Design review of the part built by this model. Coordinates are the model's own, in mm. Coordinates: 2 decimals unless noted, no trailing zeros. Write each loop counter-clockwise with the first axis right and the second up, starting at its lowest first coordinate (ties: lowest second). Pieces come first, ordered by that corner, then holes.
Solid Edge part; units mm, degrees
sketch "Sketch1" plane through (0, 0, 0) normal (0, -1, 0) x (1, 0, 0)
  line L0 (-7.62, -8.0821) -> (-7.62, -17.3179)
  line L1 (-7.62, -17.3179) -> (-12.7, -17.3179)
  line L2 (-12.7, -17.3179) -> (-12.7, -25.4)
  line L3 (-12.7, -25.4) -> (-4.6179, -25.4)
  line L4 (-4.6179, -20.32) -> (-4.6179, -25.4)
  line L5 (4.6179, -20.32) -> (-4.6179, -20.32)
  line L6 (4.6179, -25.4) -> (4.6179, -20.32)
  line L7 (4.6179, -25.4) -> (12.7, -25.4)
  line L8 (12.7, -25.4) -> (12.7, -17.3179)
  line L9 (12.7, -17.3179) -> (7.62, -17.3179)
  line L10 (7.62, -17.3179) -> (7.62, -8.0821)
  line L11 (7.62, -8.0821) -> (12.7, -8.0821)
  line L12 (12.7, -8.0821) -> (12.7, 0)
  line L13 (12.7, 8.0821) -> (12.7, 0)
  line L14 (7.62, 8.0821) -> (12.7, 8.0821)
  line L15 (7.62, 17.3179) -> (7.62, 8.0821)
  line L16 (12.7, 17.3179) -> (7.62, 17.3179)
  line L17 (12.7, 25.4) -> (12.7, 17.3179)
  line L18 (4.6179, 25.4) -> (12.7, 25.4)
  line L19 (4.6179, 25.4) -> (4.6179, 20.32)
  line L20 (4.6179, 20.32) -> (-4.6179, 20.32)
  line L21 (-4.6179, 20.32) -> (-4.6179, 25.4)
  line L22 (-12.7, 25.4) -> (-4.6179, 25.4)
  line L23 (-12.7, 17.3179) -> (-12.7, 25.4)
  line L24 (-7.62, 17.3179) -> (-12.7, 17.3179)
  line L25 (-7.62, 8.0821) -> (-7.62, 17.3179)
  line L26 (-12.7, 8.0821) -> (-7.62, 8.0821)
  line L27 (-12.7, 0) -> (-12.7, 8.0821)
  line L28 (-12.7, 0) -> (-12.7, -8.0821)
  line L29 (-12.7, -8.0821) -> (-7.62, -8.0821)
extrude "Protrusion1" add sketch "Sketch1" against normal blind 914.4
(1) Insertion check: pin 1 Ø8 at (x, y) = (1, 200.5) entering from -Z; pin 2 Ø4 at (y, z) = (677.5, 14.5) entering from -X; pin 3 Ø4.5 at (x, y) = (-0.5, 336.5) entering from +Z; pin 4 Ø3 at (x, y) = (0, 576.5) entering from -Z. Each pin has a flat end and moves straight along its axis. Give the tip position at first contact, or say it passes through.
(2) Consider section A-A (y = 755). Give the boundary of the cut face in (x, z), plus the area to 3 significant figures.
(3) Wall thickness on line 1 (Z direction, x = -8, y = 424); line 2 (X direction, y = 90.5, z = -22); line 3 (X direction, y = 860.5, z = 13): over which ranges is each line inside the solid? List them lowest first.
Results:
1. pin 1: stops at z = -25.4
1. pin 2: stops at x = -7.62
1. pin 3: stops at z = 20.32
1. pin 4: stops at z = -20.32
2. outline: (-12.7, -25.4) - (-4.62, -25.4) - (-4.62, -20.32) - (4.62, -20.32) - (4.62, -25.4) - (12.7, -25.4) - (12.7, -17.32) - (7.62, -17.32) - (7.62, -8.08) - (12.7, -8.08) - (12.7, 8.08) - (7.62, 8.08) - (7.62, 17.32) - (12.7, 17.32) - (12.7, 25.4) - (4.62, 25.4) - (4.62, 20.32) - (-4.62, 20.32) - (-4.62, 25.4) - (-12.7, 25.4) - (-12.7, 17.32) - (-7.62, 17.32) - (-7.62, 8.08) - (-12.7, 8.08) - (-12.7, -8.08) - (-7.62, -8.08) - (-7.62, -17.32) - (-12.7, -17.32) - close
2. area: 1,010 mm2
3. line 1: z = -25.4 to -17.32, -8.08 to 8.08, 17.32 to 25.4
3. line 2: x = -12.7 to -4.62, 4.62 to 12.7
3. line 3: x = -7.62 to 7.62
